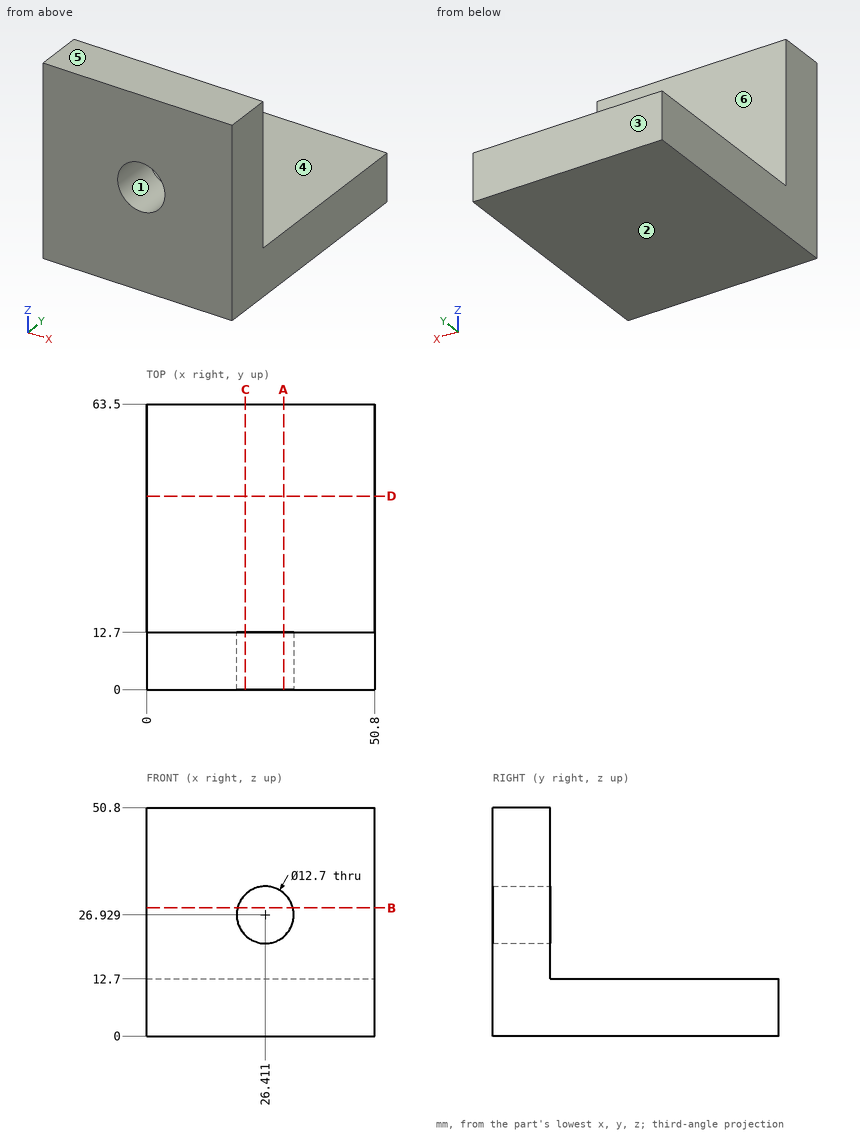
Could you check a few things on this drawing? It's one solid part, dimensions in mm from its lowest x, y, z. A direction names the side the tool comes from. Coordinates: 2 decimals unless noted, no trailing zeros. Loops run counter-clockwise (first coordinate to the right, second up) from the corner with the lowest first, then second, coordinate; pieces in that order, holes last.
1. I need wall thicknesses on L1, parallel to Y at x = 25, z = 19; L2, parallel to X at y = 3.5, z = 28.5. Which ranges of each line are inside material? Lowest first, please.
2. Imagine slicing it at A-A (x = 30.5). Please give me the cut outline in (y, z), and give its area (3 significant figures).
3. For P1, Ø10, axis at y = 35, z = 16.5, coming from the +X side; P2, Ø14.5, axis at x = 26.41, z = 26.93, coming from the +Y side, each with a flat end and sliding along its axis, tell me the tip position at first contact or that it passes through.
4. Imagine slicing it at D-D (y = 43). Please give me the cut outline in (x, z).
5. For the marked faces 5 and 6, which set-ups out of +Z, -Z, +X, -X, +Y, -Y let a thin tool reach every point of the face, with its end or its side?
6. Imagine slicing it at C-C (x = 22). Please give me the cut outline in (y, z), and give its area (3 significant figures).
7. We'd pull the mould along Z, two halves only. Please class the marked faces 1, 2, 3 and 4: released by +Z, released by -Z, zero draft, split by the parting line, or undercut.
8. Imagine slicing it at B-B (z = 28.5). Please give me the cut outline in (x, y), and give its area (3 significant figures).
Computed values:
1. L1: y = 0 to 12.7
1. L2: x = 0 to 20.26, 32.56 to 50.8
2. outline: (0, 0) - (63.5, 0) - (63.5, 12.7) - (12.7, 12.7) - (12.7, 22.07) - (0, 22.07) - close; (0, 31.79) - (12.7, 31.79) - (12.7, 50.8) - (0, 50.8) - close
2. area: 1,170 mm2
3. P1: stops at x = 50.8
3. P2: stops at y = 12.7
4. outline: (0, 0) - (50.8, 0) - (50.8, 12.7) - (0, 12.7) - close
5. face 5: +Z, +X, -X, +Y, -Y
5. face 6: +Z, +X, -X, +Y
6. outline: (0, 0) - (63.5, 0) - (63.5, 12.7) - (12.7, 12.7) - (12.7, 22.36) - (0, 22.36) - close; (0, 31.5) - (12.7, 31.5) - (12.7, 50.8) - (0, 50.8) - close
6. area: 1,170 mm2
7. face 1: undercut
7. face 2: released by -Z
7. face 3: zero draft
7. face 4: released by +Z
8. outline: (0, 0) - (20.26, 0) - (20.26, 12.7) - (0, 12.7) - close; (32.56, 0) - (50.8, 0) - (50.8, 12.7) - (32.56, 12.7) - close
8. area: 489 mm2
